from build123d import *

# Parameters (mm, degrees)
F0_R     = 12.7
F1_DEPTH = 101.6
F2_SIZE  = 2.54
F3_R     = 19.05
F3_R_2   = 12.7
F4_DEPTH = 25.4
F5_SIZE  = 0.508


with BuildPart() as f1:
    # F0 (on Top) → F1 (new body, symmetric)
    with BuildSketch(Plane.XY):
        Circle(F0_R)
    extrude(amount=F1_DEPTH, both=True)

    # F2
    f2_edges = [f1.edges().sort_by_distance(p)[0] for p in [
        (-12.7, 0, -101.6),
    ]]
    chamfer(f2_edges, length=F2_SIZE)

    # F3 (on face) → F4 (join)
    with BuildSketch(Plane.XY.offset(101.6)):
        Circle(F3_R)
        Circle(F3_R_2, mode=Mode.SUBTRACT)
        Circle(F3_R_2)
    extrude(amount=F4_DEPTH)

    # F5
    f5_edges = [f1.edges().sort_by_distance(p)[0] for p in [
        (-19.05, 0, 127),
        (-19.05, 0, 101.6),
    ]]
    chamfer(f5_edges, length=F5_SIZE)


solid = f1.part
Could you check a few things on this model? Use its own coordinates, in mm. A direction names the side the tool comes from. Round coordinates to 2 decimals unless told otherwise and drop trailing zeros. Write each loop counter-clockwise with the first axis right and the second up, starting at its lowest first coordinate (ties: lowest second). Pieces come first, ordered by that corner, then holes. Notation, with made-up numbers: (-6, 23.5) - (27, 23.5) arc R15 cw to (27, 42.5) - close; hole circle Ø2 at (2.25, 80). An arc over 180 degrees is marked (long way). Use a Markdown table: item, result.
Q1. For faces 1 (the cylindrical face through (-2.75, -12.4, 2.67)), 2 (the flat face through (0, 0, -101.6)), which set-ups out of +Z, -Z, +X, -X, +Y, -Y let a thin tool reach every point of the face, with its end or its side?
Output values:
| item | result |
|---|---|
| face 1 | -Z |
| face 2 | -Z, +X, -X, +Y, -Y |
Q2. For pin 1 (4 mm diameter, centred on x = 13, z = 12.5, fed in from -Y); pin 2 (5 mm diameter, centred on x = -7.5, z = 19.5, fed in from -Y); pin 3 (6 mm diameter, centred on y = -6.5, z = 15, fed in from +X), each with a flat end and sliding along its axis, tell me the tip position at first contact or that it passes through.
Output values:
| item | result |
|---|---|
| pin 1 | y = -6.35 |
| pin 2 | y = -11.67 |
| pin 3 | x = 12.21 |
Q3. I want a section at C-C (z = 49). List the corners of the cut face in (x, y) for me.
Output values:
| item | result |
|---|---|
| outline | circle Ø25.4 at (0, 0) |
Q4. Please list where these lines run through material, in increasing order: L1, parallel to Z at x = -3.5, y = 16; L2, parallel to Y at x = 0.5, z = 17; L3, parallel to Y at x = 4, z = 54.5.
Output values:
| item | result |
|---|---|
| L1 | 101.6 to 127 |
| L2 | -12.69 to 12.69 |
| L3 | -12.05 to 12.05 |
Q5. I want a section at A-A (y = 0). List the corners of the cut face in (x, z) for me.
Output values:
| item | result |
|---|---|
| outline | (-19.05, 102.11) - (-18.54, 101.6) - (-12.7, 101.6) - (-12.7, -99.06) - (-10.16, -101.6) - (10.16, -101.6) - (12.7, -99.06) - (12.7, 101.6) - (18.54, 101.6) - (19.05, 102.11) - (19.05, 126.49) - (18.54, 127) - (-18.54, 127) - (-19.05, 126.49) - close |
